Input: part model. Units: mm. Frame: model coordinates. A direction names the side the tool comes from. Give positions to 0.01 mm unless a question says otherwise; leave off trailing zeros. Order: outer loops, then holes, each group sorted by start corner. A loop starts at its lowest first (then second) coordinate and runs counter-clockwise, first axis right, second up. Notation, with made-up numbers: M -4,26 L 39,26 A16 cw 39,33 Z; hole C 14,33.5 d9. An arc over 180 degrees is marked long. Use a Markdown table: item, result.
from build123d import *

# Parameters (mm, degrees)
BOSS_EXTRUDE1_DEPTH = 260
REVOLVE1_ANGLE      = 90
REVOLVE2_ANGLE      = 90
SKETCH5_W           = 323.946027299
SKETCH5_H           = 266
CUT_EXTRUDE1_DEPTH  = 5
SKETCH6_W           = 350
SKETCH6_H           = 550
BOSS_EXTRUDE2_DEPTH = 5
FILLET1_R           = 5


with BuildPart() as part:
    # Sketch1 → Boss-Extrude1 (new body)
    with BuildSketch(Plane(origin=(0, 0, 0), x_dir=(1, 0, 0), z_dir=(0, 1, 0))):
        with BuildLine():
            Line((0, 0), (330, 0))
            Line((330, 0), (340, 0))
            Line((340, 0), (340, 5))
            Line((340, 5), (332.966161109, 5))
            ThreePointArc((332.966161109, 5), (330.868901888, 5.854888404), (329.966924392, 7.932330827))
            ThreePointArc((329.966924392, 7.932330827), (290.881232915, 97.954835828), (200, 135))
            Line((200, 135), (130, 135))
            ThreePointArc((130, 135), (39.118767085, 97.954835828), (0.033075608, 7.932330827))
            ThreePointArc((0.033075608, 7.932330827), (-0.868901888, 5.854888404), (-2.966161109, 5))
            Line((-2.966161109, 5), (-10, 5))
            Line((-10, 5), (-10, 0))
            Line((-10, 0), (0, 0))
        make_face()
        with BuildLine():
            Line((0.350463682, 3), (329.649536318, 3))
            ThreePointArc((329.649536318, 3), (327.711734691, 5.103277193), (326.967687675, 7.864661654))
            ThreePointArc((326.967687675, 7.864661654), (288.783973694, 95.809724232), (200, 132))
            Line((200, 132), (130, 132))
            ThreePointArc((130, 132), (41.216026306, 95.809724232), (3.032312325, 7.864661654))
            ThreePointArc((3.032312325, 7.864661654), (2.288265309, 5.103277193), (0.350463682, 3))
        make_face(mode=Mode.SUBTRACT)
    extrude(amount=BOSS_EXTRUDE1_DEPTH)

    # Sketch3 → Revolve1 (revolve)
    with BuildSketch(Plane.XZ):
        with BuildLine():
            Line((0, 0), (330, 0))
            Line((330, 0), (340, 0))
            Line((340, 0), (340, -5))
            Line((340, -5), (332.966161109, -5))
            ThreePointArc((332.966161109, -5), (330.868901888, -5.854888404), (329.966924392, -7.932330827))
            ThreePointArc((329.966924392, -7.932330827), (290.881232915, -97.954835828), (200, -135))
            Line((200, -135), (130, -135))
            ThreePointArc((130, -135), (39.118767085, -97.954835828), (0.033075608, -7.932330827))
            ThreePointArc((0.033075608, -7.932330827), (-0.868901888, -5.854888404), (-2.966161109, -5))
            Line((-2.966161109, -5), (-10, -5))
            Line((-10, -5), (-10, 0))
            Line((-10, 0), (0, 0))
        make_face()
        with BuildLine():
            Line((130, -132), (200, -132))
            ThreePointArc((200, -132), (288.783973694, -95.809724232), (326.967687675, -7.864661654))
            ThreePointArc((326.967687675, -7.864661654), (327.711734691, -5.103277193), (329.649536318, -3))
            Line((329.649536318, -3), (0.350463682, -3))
            ThreePointArc((0.350463682, -3), (2.288265309, -5.103277193), (3.032312325, -7.864661654))
            ThreePointArc((3.032312325, -7.864661654), (41.216026306, -95.809724232), (130, -132))
        make_face(mode=Mode.SUBTRACT)
    revolve(axis=Axis((0, 0, 0), (-1, 0, 0)), revolution_arc=REVOLVE1_ANGLE)

    # Sketch4 → Revolve2 (revolve)
    with BuildSketch(Plane(origin=(0, 260, 0), x_dir=(1, 0, 0), z_dir=(0, 1, 0))):
        with BuildLine():
            Line((0, 0), (330, 0))
            Line((330, 0), (340, 0))
            Line((340, 0), (340, 5))
            Line((340, 5), (332.966161109, 5))
            ThreePointArc((332.966161109, 5), (330.868901888, 5.854888404), (329.966924392, 7.932330827))
            ThreePointArc((329.966924392, 7.932330827), (290.881232915, 97.954835828), (200, 135))
            Line((200, 135), (130, 135))
            ThreePointArc((130, 135), (39.118767085, 97.954835828), (0.033075608, 7.932330827))
            ThreePointArc((0.033075608, 7.932330827), (-0.868901888, 5.854888404), (-2.966161109, 5))
            Line((-2.966161109, 5), (-10, 5))
            Line((-10, 5), (-10, 0))
            Line((-10, 0), (0, 0))
        make_face()
        with BuildLine():
            Line((0.350463682, 3), (329.649536318, 3))
            ThreePointArc((329.649536318, 3), (327.711734691, 5.103277193), (326.967687675, 7.864661654))
            ThreePointArc((326.967687675, 7.864661654), (288.783973694, 95.809724232), (200, 132))
            Line((200, 132), (130, 132))
            ThreePointArc((130, 132), (41.216026306, 95.809724232), (3.032312325, 7.864661654))
            ThreePointArc((3.032312325, 7.864661654), (2.288265309, 5.103277193), (0.350463682, 3))
        make_face(mode=Mode.SUBTRACT)
    revolve(axis=Axis((0, 260, 0), (1, 0, 0)), revolution_arc=REVOLVE2_ANGLE)

    # Sketch5 → Cut-Extrude1 (cut)
    with BuildSketch(Plane.XY):
        with Locations((164.994674026, 130)):
            Rectangle(SKETCH5_W, SKETCH5_H)
    extrude(amount=-CUT_EXTRUDE1_DEPTH, mode=Mode.SUBTRACT)

    # Sketch6 → Boss-Extrude2 (add)
    with BuildSketch(Plane.XY):
        with Locations((165, 130)):
            Rectangle(SKETCH6_W, SKETCH6_H)
        with BuildLine():
            Line((133, -135.00977849), (197, -135.00977849))
            ThreePointArc((197, -135.00977849), (291.045201898, -96.054980388), (330, -2.00977849))
            Line((330, -2.00977849), (330, 262.00977849))
            ThreePointArc((330, 262.00977849), (291.045201898, 356.054980388), (197, 395.00977849))
            Line((197, 395.00977849), (133, 395.00977849))
            ThreePointArc((133, 395.00977849), (38.954798102, 356.054980388), (0, 262.00977849))
            Line((0, 262.00977849), (0, -2.00977849))
            ThreePointArc((0, -2.00977849), (38.954798102, -96.054980388), (133, -135.00977849))
        make_face(mode=Mode.SUBTRACT)
    extrude(amount=BOSS_EXTRUDE2_DEPTH)

    # Fillet1
    fillet1_edges = [part.edges().sort_by_distance(p)[0] for p in [
        (340, -145, 2.5),
        (340, 405, 2.5),
        (-10, 405, 2.5),
        (-10, -145, 2.5),
    ]]
    fillet(fillet1_edges, radius=FILLET1_R)


solid = part.part
1) Cut plane B-B on y = 18. Return loops of the section in (x, z).
Response values:
| item | result |
|---|---|
| outline | M -10,-5 L -2.97,-5 A3 cw 0.03,-7.93 A130 ccw 130,-135 L 200,-135 A130 ccw 329.97,-7.93 A3 cw 332.97,-5 L 340,-5 L 340,5 L 330,5 L 330,0 L 326.97,0 L 326.97,-3 L 329.65,-3 A6 ccw 326.97,-7.86 A127 cw 200,-132 L 130,-132 A127 cw 3.03,-7.86 A6 ccw 0.35,-3 L 3.02,-3 L 3.02,0 L 0,0 L 0,5 L -10,5 Z |
2) First-contact query: pin 1 Ø21 at (x, y) = (180.5, 173) entering from +Z; pin 2 Ø1 at (y, z) = (105.5, -21.5) entering from +X; pin 3 Ø1.5 at (x, z) = (236.5, -73) entering from +Y. Flat tips, straight axial feed; report the tip coordinate or a pass-through.
Response values:
| item | result |
|---|---|
| pin 1 | stops at z = -132 |
| pin 2 | stops at x = 329.01 |
| pin 3 | stops at y = 367.86 |
3) Cut plane A-A on x = 147. Return loops of the section in (y, z).
Response values:
| item | result |
|---|---|
| outline | M -145,0 L -135.01,0 L -135.01,5 L -145,5 Z; M -135,0 A135 ccw 0,-135 L 260,-135 A135 ccw 395,0 L 392,0 A132 cw 260,-132 L 0,-132 A132 cw -132,0 Z; M 395.01,0 L 405,0 L 405,5 L 395.01,5 Z |
4) Material intervals for line 1 (Y direction, x = 239, z = -93); line 2 (Y direction, x = 65, z = -84); line 3 (X direction, y = 157, z = -106.5), sorted ascending. Write a range as from..to.
Response values:
| item | result |
|---|---|
| line 1 | y = -89.42..-84.81, 344.81..349.42 |
| line 2 | y = -82.28..-77.23, 337.23..342.28 |
| line 3 | x = 48.77..53.67, 276.33..281.23 |
5) Reachability of faces 1 (the face through (164, -142, 0)), 2 (the face through (40.131, 128.18, -98.934)), 3 (the face through (292.07, 355.02, 2.46)), 4 (the face through (164, 398, 0)) from +Z, -Z, +X, -X, +Y, -Y: full face, straight path, thin tool, end or side. Return the list, or none.
Response values:
| item | result |
|---|---|
| face 1 | -Z, -Y |
| face 2 | -Z, -X, +Y, -Y |
| face 3 | +Z |
| face 4 | -Z, +Y |
